The listing builds one solid part. Answer for the finished solid, in the listing's coordinates (mm). Round coordinates to 2 decimals unless told otherwise and drop trailing zeros. Loops run counter-clockwise (first coordinate to the right, second up) from the corner with the lowest first, then second, coordinate; pieces in that order, holes last. Notation, with made-up numbers: (45, -27.5) -> (89, -27.5) arc R24 ccw to (89, 8.5) -> close; hole circle Ø3 at (40, 10). An arc over 180 degrees is marked (long way). Use a Markdown table: item, result. Add a question column.
Q1. Section D-D on x = 1 is taken. Give the vertices of the cut face in (y, z), then the cut area to 3 significant figures.
Q2. Given pin 1 Ø0.8 at (x, z) = (-6.5, 1) entering from -Y, flat-ended and moving along its own axis, determine where the tip first touches the part or whether it passes through.
Q3. Consider line 1 (Y direction, x = -24.8, z = 0.9); line 2 (Y direction, x = 15.5, z = 1.3); line 3 (Y direction, x = -2, z = 0.7). Determine where each line is inside the solid, lowest interval first.
Q4. Section B-B on z = 1.1 is taken. Give the number of separate pieces and of enclosed holes in the cut face, then the cut area to 3 significant figures.
Q5. Section C-C on y = -38.3 is taken. Give the vertices of the cut face in (x, z).
Q6. Section A-A on x = -24.8 is taken. Give the vertices of the cut face in (y, z), then the cut area to 3 significant figures.
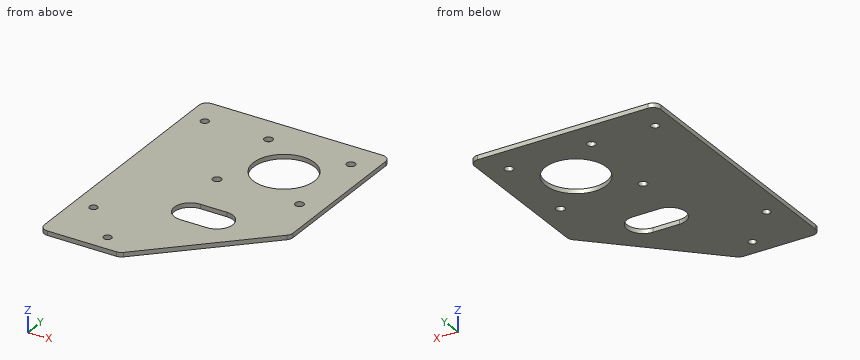
Autodesk Inventor part; units mm, degrees
ref_plane "YZ Plane" through (0, 0, 0) normal (1, 0, 0) x (0, 1, 0)
ref_plane "XZ Plane" through (0, 0, 0) normal (0, 1, 0) x (-1, 0, 0)
ref_plane "XY Plane" through (0, 0, 0) normal (0, 0, 1) x (1, 0, 0)
sketch "Эскиз1" plane through (0, 0, 0) normal (0, 0, 1) x (1, 0, 0)
  line L0 (15.5, 15.5) -> (-15.5, 15.5) construction
  line L1 (-15.5, 15.5) -> (-15.5, -15.5) construction
  line L2 (-15.5, -15.5) -> (15.5, -15.5) construction
  line L3 (15.5, -15.5) -> (15.5, 15.5) construction
  line L4 (15.5, 15.5) -> (-15.5, -15.5) construction
  line L5 (-15.5, 15.5) -> (15.5, -15.5) construction
  circle A0 centre (-15.5, 15.5) radius 1.6
  circle A1 centre (15.5, 15.5) radius 1.6
  circle A2 centre (15.5, -15.5) radius 1.6
  circle A3 centre (-15.5, -15.5) radius 1.6
  circle A4 centre (0, 0) radius 11.5
  line L6 (-46.3, 25.9) -> (23.9, 25.9)
  line L7 (23.9, 25.9) -> (23.9, -34.1)
  line L8 (-16.1, -73.1) -> (-46.3, -73.1)
  line L9 (-46.3, -73.1) -> (-46.3, 25.9)
  line L10 (-16.1, -73.1) -> (23.9, -34.1)
  line L11 (-11.3, -38.3) -> (-1.3, -38.3) construction
  line L12 (-11.3, -32.3) -> (-1.3, -32.3)
  line L13 (-1.3, -44.3) -> (-11.3, -44.3)
  arc A5 (-11.3, -32.3) -> (-11.3, -44.3) centre (-11.3, -38.3) ccw
  arc A6 (-1.3, -44.3) -> (-1.3, -32.3) centre (-1.3, -38.3) ccw
  circle A7 centre (-39.1, 14.9) radius 1.5
  circle A8 centre (-39.1, -52.1) radius 1.5
  circle A9 centre (-24.8, -66.5) radius 1.5
  point P0 (-6.3, -38.3)
  dimension "d0" = 31
  dimension "d1" = 31
  dimension "d2" = 3.2
  dimension "d3" = 3.2
  dimension "d4" = 3.2
  dimension "d5" = 3.2
  dimension "d6" = 23
  dimension "d7" = 6.8
  dimension "d8" = 8.4
  dimension "d9" = 8.8
  dimension "d10" = 70.2
  dimension "d11" = 60
  dimension "d12" = 99
  dimension "d13" = 40
  dimension "d14" = 22
  dimension "d15" = 12
  dimension "d16" = 20.8
  dimension "d17" = 29
  dimension "d18" = 3
  dimension "d19" = 3
  dimension "d20" = 7.2
  dimension "d21" = 7.2
  dimension "d22" = 67
  dimension "d23" = 21
  dimension "d24" = 58.2
  dimension "d25" = 3
  dimension "d26" = 21.5
  dimension "d27" = 6.6
extrude "Выдавливание1" add sketch "Эскиз1" along normal blind 1.65
fillet "Сопряжение1" radius 3 5 edges at (23.9, 25.9, 0.825) (-46.3, 25.9, 0.825) (23.9, -34.1, 0.825) (-16.1, -73.1, 0.825) (-46.3, -73.1, 0.825)
properties part number "пластина  экструдера"
Checked values:
| question | item | result |
|---|---|---|
| 1 | outline | (-56.43, 0) -> (-43.84, 0) -> (-43.84, 1.65) -> (-56.43, 1.65) -> close; (-32.76, 0) -> (-11.46, 0) -> (-11.46, 1.65) -> (-32.76, 1.65) -> close; (11.46, 0) -> (25.9, 0) -> (25.9, 1.65) -> (11.46, 1.65) -> close |
| 1 | area | 79.7 mm2 |
| 2 | pin 1 | stops at y = -64.13 |
| 3 | line 1 | y = -73.1 to -68, -65 to 25.9 |
| 3 | line 2 | y = -42.29 to -17.1, -13.9 to 13.9, 17.1 to 25.9 |
| 3 | line 3 | y = -59.35 to -44.3, -32.3 to -11.32, 11.32 to 25.9 |
| 4 | separate pieces | 1 |
| 4 | enclosed holes | 9 |
| 4 | area | 5,460 mm2 |
| 5 | outline | (-46.3, 0) -> (-17.3, 0) -> (-17.3, 1.65) -> (-46.3, 1.65) -> close; (4.7, 0) -> (19.59, 0) -> (19.59, 1.65) -> (4.7, 1.65) -> close |
| 6 | outline | (-73.1, 0) -> (-68, 0) -> (-68, 1.65) -> (-73.1, 1.65) -> close; (-65, 0) -> (25.9, 0) -> (25.9, 1.65) -> (-65, 1.65) -> close |
| 6 | area | 158 mm2 |
